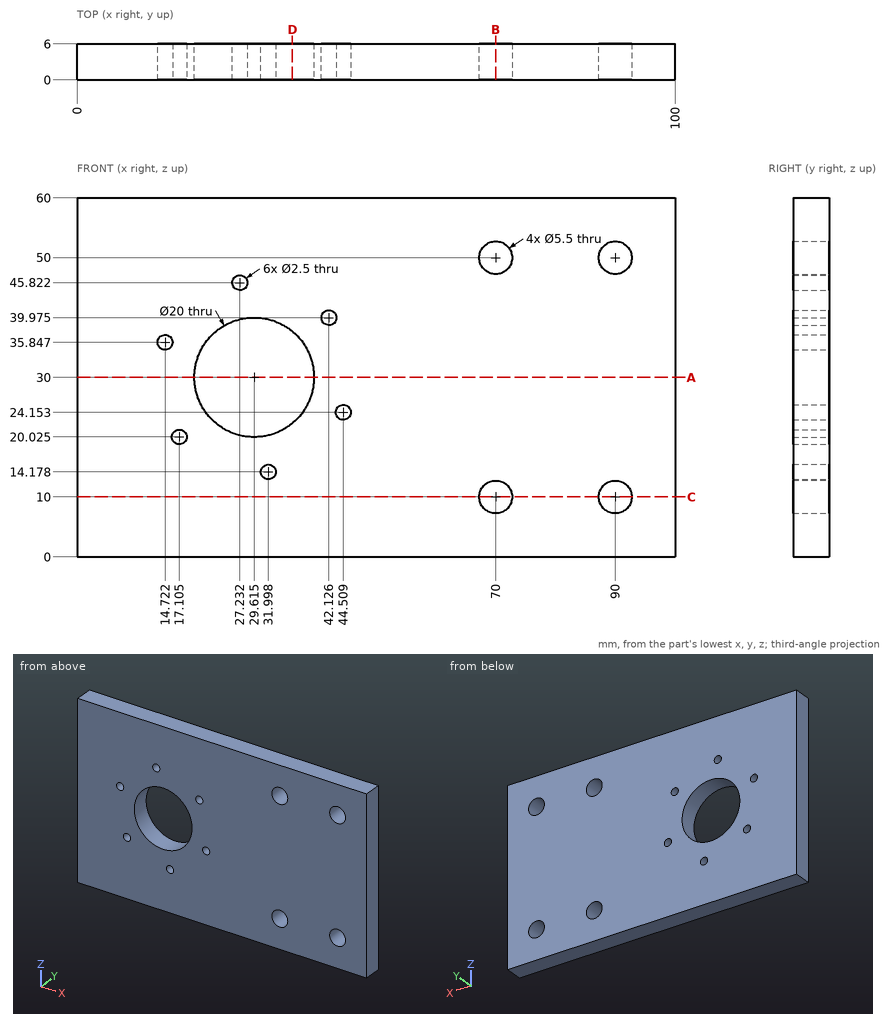
For this review, use the dimensioned drawing (mm, ordinates from the lowest corner) and the shaded views. Round coordinates to 2 decimals unless told otherwise and drop trailing zeros. Order: outer loops, then holes, each group sorted by start corner. A loop starts at its lowest first (then second) coordinate and runs counter-clockwise, first axis right, second up. Notation, with made-up numbers: M 6.5,-15 L 40.5,-15 A20 ccw 40.5,16 Z; hole C 63,78.25 d11. An arc over 180 degrees is marked long. Use a Markdown table: item, result. Add a question column.
Item 1: To check wall thickness, follow line 1 along X through (y, z) = (2.7, 50); line 2 along Z through (x, y) = (90, 3.45); line 3 along X through (y, z) = (1.4, 30) (1 decimal). State the ranges of each line that lie inside material, in increasing order.
Item 2: Add section C-C, the plane z = 10. Give the boundary of the cut face in (x, y).
Item 3: Add section B-B, the plane x = 70. Give the boundary of the cut face in (y, z).
Item 4: Add section D-D, the plane x = 36. Give the boundary of the cut face in (y, z), then the cut area to 3 significant figures.
Item 5: Add section A-A, the plane z = 30. Give the boundary of the cut face in (x, y) (1 decimal), then the cut area to 3 significant figures.
Geometry results:
| question | item | result |
|---|---|---|
| 1 | line 1 | x = 0 to 67.25, 72.75 to 87.25, 92.75 to 100 |
| 1 | line 2 | z = 0 to 7.25, 12.75 to 47.25, 52.75 to 60 |
| 1 | line 3 | x = 0 to 19.6, 39.6 to 100 |
| 2 | outline | M 0,0 L 67.25,0 L 67.25,6 L 0,6 Z; M 72.75,0 L 87.25,0 L 87.25,6 L 72.75,6 Z; M 92.75,0 L 100,0 L 100,6 L 92.75,6 Z |
| 3 | outline | M 0,0 L 6,0 L 6,7.25 L 0,7.25 Z; M 0,12.75 L 6,12.75 L 6,47.25 L 0,47.25 Z; M 0,52.75 L 6,52.75 L 6,60 L 0,60 Z |
| 4 | outline | M 0,0 L 6,0 L 6,22.3 L 0,22.3 Z; M 0,37.7 L 6,37.7 L 6,60 L 0,60 Z |
| 4 | area | 268 mm² |
| 5 | outline | M 0,0 L 19.6,0 L 19.6,6 L 0,6 Z; M 39.6,0 L 100,0 L 100,6 L 39.6,6 Z |
| 5 | area | 480 mm² |
